```python
from build123d import *

# Parameters (mm, degrees)
F2_DEPTH  = 600
F3_R      = 50
F4_DEPTH  = 600
F5_R      = 50
F6_DEPTH  = 300
F7_R      = 50
F8_DEPTH  = 300
F9_R      = 30
F10_DEPTH = 600.001
F11_R     = 15
F12_DEPTH = 25


with BuildPart() as f2:
    # F1 (on Front) → F2 (new body)
    with BuildSketch(Plane.XZ):
        Polygon((-579.289322, -1398.528137), (-600, -1448.528137), (600, -1448.528137), (579.289322, -1398.528137), align=None)
    extrude(amount=F2_DEPTH)

    # F3 (on face) → F4 (join, through all)
    with BuildSketch(Plane.XZ):
        with Locations((-600, -1448.528137)):
            Circle(F3_R)
        with Locations((600, -1448.528137)):
            Circle(F3_R)
    extrude(amount=F4_DEPTH)

    # F5 (on Front) → F6 (cut, symmetric)
    with BuildSketch(Plane.XZ):
        with Locations((600, -1448.528137)):
            Circle(F5_R)
    extrude(amount=F6_DEPTH, both=True, mode=Mode.SUBTRACT)

    # F7 (on face) → F8 (cut, through all)
    with BuildSketch(Plane.XZ.offset(600)):
        with Locations((-600, -1448.528137)):
            Circle(F7_R)
    extrude(amount=-F8_DEPTH, mode=Mode.SUBTRACT)

    # F9 (on Front) → F10 (cut, through all)
    with BuildSketch(Plane.XZ):
        with Locations((-600, -1448.528137)):
            Circle(F9_R)
        with Locations((600, -1448.528137)):
            Circle(F9_R)
    extrude(amount=F10_DEPTH, mode=Mode.SUBTRACT)

    # F11 (on face) → F12 (join)
    with BuildSketch(Plane.XZ.offset(600)):
        Polygon((141.553584, -498.528137), (-141.553584, -498.528137), (-514.34579, -1398.528137), (514.34579, -1398.528137), align=None)
        with BuildLine():
            Line((-336.048902, -1229.393966), (-82.406747, -617.047634))
            ThreePointArc((-82.406747, -617.047634), (-71.357468, -603.584049), (-54.690361, -598.528137))
            Line((-54.690361, -598.528137), (54.690361, -598.528137))
            ThreePointArc((54.690361, -598.528137), (71.357468, -603.584049), (82.406747, -617.047634))
            Line((82.406747, -617.047634), (336.048902, -1229.393966))
            ThreePointArc((336.048902, -1229.393966), (331.428406, -1276.306649), (289.854925, -1298.528137))
            Line((289.854925, -1298.528137), (-289.854925, -1298.528137))
            ThreePointArc((-289.854925, -1298.528137), (-331.428406, -1276.306649), (-336.048902, -1229.393966))
        make_face(mode=Mode.SUBTRACT)
        with Locations((-110, -598.528137)):
            Circle(F11_R, mode=Mode.SUBTRACT)
        with Locations((110, -598.528137)):
            Circle(F11_R, mode=Mode.SUBTRACT)
    extrude(amount=-F12_DEPTH)

    # F13: F2 across plane


with BuildPart() as f2_1:
    add(f2.part)
    add(f2.part.mirror(Plane.XZ))


solid = f2_1.part
```
Check sheet for the modelled part. Datum: model origin and axes. Units: mm. A direction names the side the tool comes from. Give positions to 0.01 mm unless a question says otherwise; leave off trailing zeros. Order: outer loops, then holes, each group sorted by start corner. A loop starts at its lowest first (then second) coordinate and runs counter-clockwise, first axis right, second up. Notation, with made-up numbers: M 55,52 L 72,52 A35 cw 72,88 Z; hole C 80.5,18.5 d11. An arc over 180 degrees is marked long. Answer in a Markdown table with one row per item.
1) Cross-section at D-D, the plane z = -646. Enter the section's corners in (x, y), plus the area to 3 significant figures.
Filled sheet:
| item | result |
|---|---|
| outline | M -202.64,-600 L -94.4,-600 L -94.4,-575 L -202.64,-575 Z; M -202.64,575 L -94.4,575 L -94.4,600 L -202.64,600 Z; M 94.4,-600 L 202.64,-600 L 202.64,-575 L 94.4,-575 Z; M 94.4,575 L 202.64,575 L 202.64,600 L 94.4,600 Z |
| area | 10,800 mm2 |
2) Thickness scan on L1, parallel to Y at x = 401, z = -1237; L2, parallel to Z at x = 110, y = 593; L3, parallel to X at y = -342, z = -1457. Record the ranges inside material, lowest first. Write a range as [from, to].
Filled sheet:
| item | result |
|---|---|
| L1 | y = [-600, -575], [575, 600] |
| L2 | z = [-1448.53, -1298.53], [-683.66, -613.53], [-583.53, -498.53] |
| L3 | x = [550.72, 571.22], [628.78, 649.28] |
3) Release check for a two-part mould opening along X. For faces 1 (the cylindrical face through (613.843, -447.9, -1475.143)), 2 (the cylindrical face through (-558.2, 452.1, -1421.09)), 3 (the flat face through (8, -8, -1398.528)), 4 (the cylindrical face through (331.81, 587.67, -1275.73)) record: +X half, -X half, draft (parallel to the pull), parting line (faces both ways), or undercut.
Filled sheet:
| item | result |
|---|---|
| face 1 | undercut |
| face 2 | -X half |
| face 3 | draft |
| face 4 | undercut |
4) Cross-section at C-C, the plane x = 600. Enter the section's corners in (y, z), plus the area to 3 significant figures.
Filled sheet:
| item | result |
|---|---|
| outline | M -600,-1498.53 L -300,-1498.53 L -300,-1478.53 L -600,-1478.53 Z; M -600,-1418.53 L -300,-1418.53 L -300,-1398.53 L -600,-1398.53 Z; M 300,-1498.53 L 600,-1498.53 L 600,-1478.53 L 300,-1478.53 Z; M 300,-1418.53 L 600,-1418.53 L 600,-1398.53 L 300,-1398.53 Z |
| area | 24,000 mm2 |
5) Cross-section at A-A, the plane x = -600. Enter the section's corners in (y, z), plus the area to 3 significant figures.
Filled sheet:
| item | result |
|---|---|
| outline | M -300,-1498.53 L 300,-1498.53 L 300,-1478.53 L -300,-1478.53 Z; M -300,-1418.53 L 300,-1418.53 L 300,-1398.53 L -300,-1398.53 Z |
| area | 24,000 mm2 |
6) Access from +Z, -Z, +X, -X, +Y, -Y to the whole of each face (thin tool, end or side, straight path). Record for faces 5 (the cylindrical face through (-331.04, -587.67, -1276.88)), 6 (the flat face through (-325.34, -587.67, -942.23)), 7 (the flat face through (-578, -300, -1470)), 8 (the flat face through (-578, 300, -1470)), 9 (the flat face through (622, 300, -1470)).
Filled sheet:
| item | result |
|---|---|
| face 5 | +Y, -Y |
| face 6 | +Z, -X, +Y, -Y |
| face 7 | -Z, -X, -Y |
| face 8 | -Z, -X, +Y |
| face 9 | -Z, +X |
7) Cross-section at B-B, the plane y = -444. Enter the section's corners in (x, z).
Filled sheet:
| item | result |
|---|---|
| outline | M -580.87,-1402.33 A50 cw -550,-1448.53 L 550,-1448.53 A50 ccw long 580.87,-1402.33 L 579.29,-1398.53 L -579.29,-1398.53 Z; hole C 600,-1448.53 d60 |
8) Gauge pin test, flat ends, axial feed: P1, Ø7.5, axis at x = 16.5, y = -582.5, coming from the -Z side; P2, Ø8, axis at x = -377, z = -1052, coming from the +Y side; P3, Ø1.5, axis at x = -439, y = 413.5, coming from the +Z side. Record the tip position at first contact, or that the pin passes through.
Filled sheet:
| item | result |
|---|---|
| P1 | stops at z = -1448.53 |
| P2 | passes through |
| P3 | stops at z = -1398.53 |
